Design review of the part built by this model. Coordinates are the model's own, in mm. A direction names the side the tool comes from. Coordinates: 2 decimals unless noted, no trailing zeros. Order: outer loops, then holes, each group sorted by start corner. A loop starts at its lowest first (then second) coordinate and runs counter-clockwise, first axis right, second up.
from build123d import *

# Parameters (mm, degrees)
BOSS_EXTRUDE1_DEPTH                               = 25.4
SKETCH2_W                                         = 12.7
SKETCH2_H                                         = 3.175
CUT_EXTRUDE1_DEPTH                                = 1.5875
CSK_FOR_6_FLAT_HEAD_MACHINE_SCREW_100_D           = 3.7973
CSK_FOR_6_FLAT_HEAD_MACHINE_SCREW_100_DEPTH       = 25.4
CSK_FOR_6_FLAT_HEAD_MACHINE_SCREW_100_CSINK_D     = 7.0866
CSK_FOR_6_FLAT_HEAD_MACHINE_SCREW_100_CSINK_ANGLE = 100
CSK_FOR_6_FLAT_HEAD_MACHINE_SCREW_100_TIP         = 1.140824014


with BuildPart() as part:
    # Sketch1 → Boss-Extrude1 (new body)
    with BuildSketch(Plane.XY):
        Polygon((-12.7, 0), (-12.7, 63.5), (25.4, 63.5), (25.4, 50.8), (0, 50.8), (0, 0), align=None)
    extrude(amount=-BOSS_EXTRUDE1_DEPTH)

    # Sketch2 → Cut-Extrude1 (cut)
    with BuildSketch(Plane(origin=(0, 0, 0), x_dir=(0, 0, -1), z_dir=(1, 0, 0))):
        with Locations((12.7, 14.2875)):
            Rectangle(SKETCH2_W, SKETCH2_H)
    extrude(amount=-CUT_EXTRUDE1_DEPTH, mode=Mode.SUBTRACT)

    # CSK for #6 Flat Head Machine Screw (100)1
    with Locations(Plane(origin=(-12.7, -5.150678534, -61.119160157), x_dir=(0, 0, 1), z_dir=(-1, 0, 0))):
        with Locations((48.419160157, 25.344845691)):
            CounterSinkHole(CSK_FOR_6_FLAT_HEAD_MACHINE_SCREW_100_D / 2, CSK_FOR_6_FLAT_HEAD_MACHINE_SCREW_100_CSINK_D / 2, depth=CSK_FOR_6_FLAT_HEAD_MACHINE_SCREW_100_DEPTH, counter_sink_angle=CSK_FOR_6_FLAT_HEAD_MACHINE_SCREW_100_CSINK_ANGLE)
            with Locations((0, 0, -(CSK_FOR_6_FLAT_HEAD_MACHINE_SCREW_100_DEPTH + CSK_FOR_6_FLAT_HEAD_MACHINE_SCREW_100_TIP / 2))):  # 118° drill point
                Cone(0, CSK_FOR_6_FLAT_HEAD_MACHINE_SCREW_100_D / 2, CSK_FOR_6_FLAT_HEAD_MACHINE_SCREW_100_TIP, mode=Mode.SUBTRACT)


solid = part.part
1. To check wall thickness, follow line 1 (Y direction, x = -4.75, z = -12.7); line 2 (X direction, y = 15, z = -17.75); line 3 (X direction, y = 39, z = -7.25). State the ranges of each line that lie inside material, in increasing order.
2. Add section A-A (z = -12.7). Give the boundary of the cut face in (x, y) (1 decimal).
3. Add section C-C (y = 34). Give the boundary of the cut face in (x, z).
4. Mouldability with a two-part tool opening along Y and no side actions: class faces 4 (the flat face through (6, 63.5, -13)), 5 (the flat face through (-1, 14, -19.05)), 6 (the flat face through (-1, 14, -6.35)), 7 (the flat face through (-2, 39, 0)) as pulls with the +Y half, pulls with the -Y half, needs draft (parallel to the pull), parting line crosses it, or undercut.
5. Add section D-D (x = 9). Give the boundary of the cut face in (y, z).
6. Add section B-B (z = -23). Give the boundary of the cut face in (x, y), and give its area (3 significant figures).
7. Insertion check: pin 1 (1 mm diameter, centred on y = 15, z = -10.5, fed in from +X); pin 2 (6 mm diameter, centred on x = 10, z = -7, fed in from -Y); pin 3 (7.5 mm diameter, centred on y = 36, z = -10, fed in from +X). Each pin has a flat end and moves straight along its axis. Give the tip position at first contact, or say it passes through.
8. For faces 1 (the cylindrical face through (-5.581, 22.077, -12.453)), 2 (the flat face through (-1.588, 14, -13)), 3 (the flat face through (0, 26, -13)), list the 3-axis set-ups (+Z, -Z, +X, -X, +Y, -Y) from which the entire face can be reached by the end or side of a thin tool; tool diameter is ignored.
Solution:
1. line 1: y = 0 to 18.3, 22.09 to 63.5
1. line 2: x = -12.7 to -1.59
1. line 3: x = -12.7 to 0
2. outline: (-12.7, 0) - (0, 0) - (0, 12.7) - (-1.6, 12.7) - (-1.6, 15.9) - (0, 15.9) - (0, 18.3) - (-11.3, 18.3) - (-12.7, 16.7) - close; (-12.7, 23.7) - (-11.3, 22.1) - (0, 22.1) - (0, 50.8) - (25.4, 50.8) - (25.4, 63.5) - (-12.7, 63.5) - close
3. outline: (-12.7, -25.4) - (0, -25.4) - (0, 0) - (-12.7, 0) - close
4. face 4: pulls with the +Y half
4. face 5: undercut
4. face 6: undercut
4. face 7: needs draft
5. outline: (50.8, -25.4) - (63.5, -25.4) - (63.5, 0) - (50.8, 0) - close
6. outline: (-12.7, 0) - (0, 0) - (0, 50.8) - (25.4, 50.8) - (25.4, 63.5) - (-12.7, 63.5) - close
6. area: 1,130 mm2
7. pin 1: stops at x = -1.59
7. pin 2: stops at y = 50.8
7. pin 3: stops at x = 0
8. face 1: +X, -X
8. face 2: +X
8. face 3: +Z, -Z, +X, -Y
